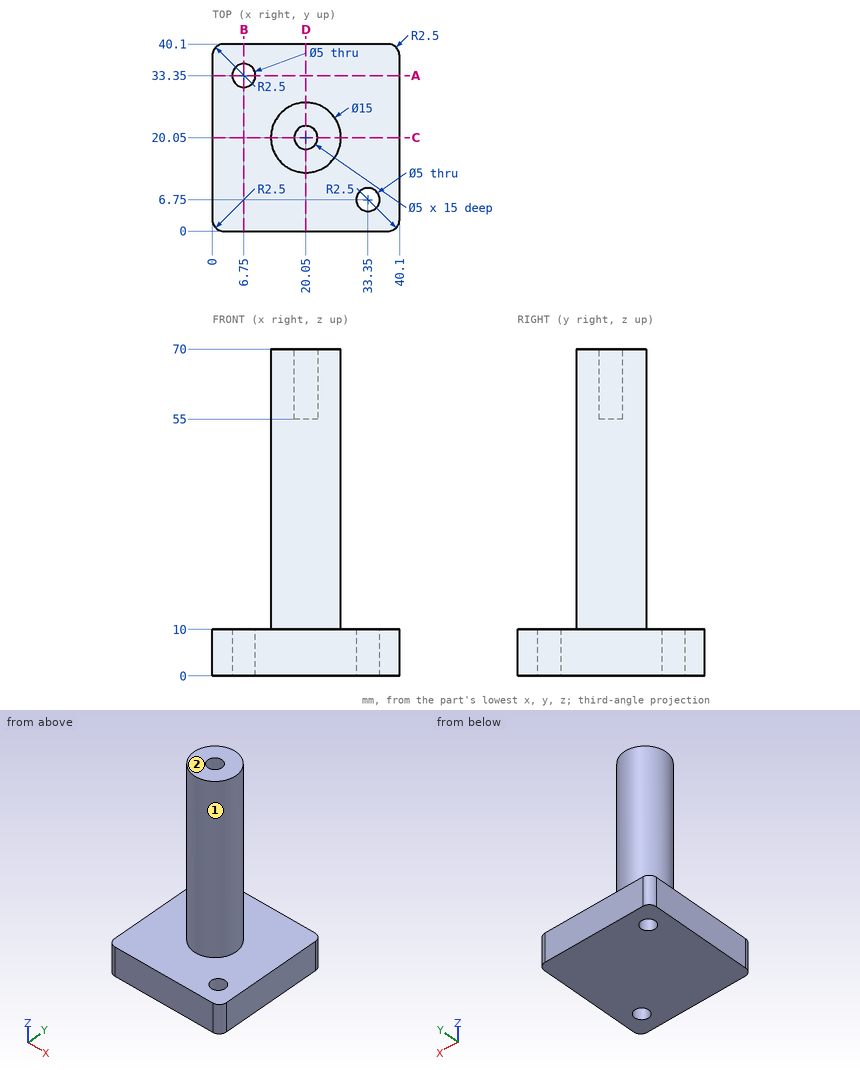
Input: dimensioned drawing with shaded views. Units: mm. Origin: part minimum x, y, z. A direction names the side the tool comes from. Coordinates: 2 decimals unless noted, no trailing zeros. Write each loop counter-clockwise with the first axis right and the second up, starting at its lowest first coordinate (ties: lowest second). Pieces come first, ordered by that corner, then holes. Notation, with made-up numbers: M -9.5,-12.75 L 2.5,-12.75 A12 cw 2.5,5.25 Z; hole C 41.25,84.25 d8. An arc over 180 degrees is marked long. Use a Markdown table: item, result.
1) Section A-A, the plane y = 33.35. Output: boundary loops of the cut face in (x, z).
Conclusion:
| item | result |
|---|---|
| outline | M 0,0 L 4.25,0 L 4.25,10 L 0,10 Z; M 9.25,0 L 40.1,0 L 40.1,10 L 9.25,10 Z |
2) First-contact query: pin 1 Ø6.5 at (x, y) = (6.75, 33.35) entering from +Z; pin 2 Ø5 at (y, z) = (20, 45) entering from +X; pin 3 Ø8 at (y, z) = (16.5, 50.5) entering from -X; pin 4 Ø3 at (x, z) = (29.5, 60) entering from -Y. Flat tips, straight axial feed; report the tip coordinate or a pass-through.
Conclusion:
| item | result |
|---|---|
| pin 1 | stops at z = 10 |
| pin 2 | stops at x = 27.55 |
| pin 3 | stops at x = 12.55 |
| pin 4 | passes through |
3) Section B-B, the plane x = 6.75. Output: boundary loops of the cut face in (y, z).
Conclusion:
| item | result |
|---|---|
| outline | M 0,0 L 30.85,0 L 30.85,10 L 0,10 Z; M 35.85,0 L 40.1,0 L 40.1,10 L 35.85,10 Z |
4) Reachability of the marked faces 1 and 2 from +Z, -Z, +X, -X, +Y, -Y: full face, straight path, thin tool, end or side. Return the list, or none.
Conclusion:
| item | result |
|---|---|
| face 1 | +Z |
| face 2 | +Z, +X, -X, +Y, -Y |
5) Section C-C, the plane y = 20.05. Output: boundary loops of the cut face in (x, z), then the cut area to 3 significant figures.
Conclusion:
| item | result |
|---|---|
| outline | M 0,0 L 40.1,0 L 40.1,10 L 27.55,10 L 27.55,70 L 22.55,70 L 22.55,55 L 17.55,55 L 17.55,70 L 12.55,70 L 12.55,10 L 0,10 Z |
| area | 1,230 mm^2 |
6) Ray query, L1, parallel to Y at x = 6.75, z = 3; L2, parallel to Y at x = 20, z = 60; L3, parallel to Z at x = 13.5, y = 2. Return the intervals inside material, ascending.
Conclusion:
| item | result |
|---|---|
| L1 | y = 0 to 30.85, 35.85 to 40.1 |
| L2 | y = 12.55 to 17.55, 22.55 to 27.55 |
| L3 | z = 0 to 10 |
